```python
from build123d import *

# Parameters (mm, degrees)
SKETCH1_W           = 152.4
SKETCH1_H           = 50.8
BOSS_EXTRUDE1_DEPTH = 6
BOSS_EXTRUDE2_DEPTH = 152.4
SKETCH7_W           = 16.51
SKETCH7_H           = 19.05
SKETCH7_R           = 2
BOSS_EXTRUDE3_DEPTH = 7
FILLET1_R           = 3.175
SKETCH8_R           = 3.025
CUT_EXTRUDE1_DEPTH  = 10


with BuildPart() as part:
    # Sketch1 → Boss-Extrude1 (new body)
    with BuildSketch(Plane.XY):
        Rectangle(SKETCH1_W, SKETCH1_H)
    extrude(amount=BOSS_EXTRUDE1_DEPTH)

    # Sketch5 → Boss-Extrude2 (add)
    with BuildSketch(Plane.ZY.offset(76.2)):
        Polygon((6, 25.4), (24.489687901, 25.4), (6, -25.4), align=None)
    extrude(amount=-BOSS_EXTRUDE2_DEPTH)

    # Sketch7 → Boss-Extrude3 (add)
    # profile 1 of 2: a face of its own
    with BuildSketch(Plane(origin=(0, 0, 0), x_dir=(-1, 0, 0), z_dir=(0, 0, -1))):
        with Locations((-84.455, 0)):
            Rectangle(SKETCH7_W, SKETCH7_H)
        with Locations((-84.455, 0)):
            Circle(SKETCH7_R, mode=Mode.SUBTRACT)
    # profile 2 of 2: a face of its own
    with BuildSketch(Plane(origin=(0, 0, 0), x_dir=(-1, 0, 0), z_dir=(0, 0, -1))):
        with Locations((84.455, 0)):
            Rectangle(SKETCH7_W, SKETCH7_H)
        with Locations((84.455, 0)):
            Circle(SKETCH7_R, mode=Mode.SUBTRACT)
    extrude(amount=-BOSS_EXTRUDE3_DEPTH)

    # Fillet1
    fillet1_edges = [part.edges().sort_by_distance(p)[0] for p in [
        (-76.2, 0, 15.24484395),
        (76.2, 0, 15.24484395),
        (0, 25.4, 24.489687901),
        (0, -25.4, 6),
        (76.2, -9.525, 3.5),
        (92.71, -9.525, 3.5),
        (92.71, 9.525, 3.5),
        (76.2, 9.525, 3.5),
        (-76.2, -9.525, 3.5),
        (-76.2, 9.525, 3.5),
        (-92.71, 9.525, 3.5),
        (-92.71, -9.525, 3.5),
        (76.2, -25.4, 3),
        (-76.2, -25.4, 3),
        (-76.2, 25.4, 12.24484395),
        (76.2, 25.4, 12.24484395),
    ]]
    fillet(fillet1_edges, radius=FILLET1_R)

    # Sketch8 → Cut-Extrude1 (cut)
    with BuildSketch(Plane(origin=(0, -4.899598401, 13.461535972), x_dir=(1, 0, 0), z_dir=(0, -0.3420201433256695, 0.9396926207859082))):
        with Locations(Location((-66.11875, 7.355813283, 0), (0, 0, 270))):
            Circle(SKETCH8_R)
        with Locations(Location((66.11875, 7.355813283, 0), (0, 0, 270))):
            Circle(SKETCH8_R)
    extrude(amount=-CUT_EXTRUDE1_DEPTH, mode=Mode.SUBTRACT)


solid = part.part
```
Could you check a few things on this model? Use its own coordinates, in mm. A direction names the side the tool comes from. Give positions to 0.01 mm unless a question says otherwise; leave off trailing zeros. Order: outer loops, then holes, each group sorted by start corner. A loop starts at its lowest first (then second) coordinate and runs counter-clockwise, first axis right, second up.
Q1. I'm going to push flat-ended pins straight in: P1, Ø5, axis at x = -84.455, y = 0, coming from the +Z side; P2, Ø3.5, axis at x = 86, z = 5, coming from the -Y side (3 decimals); P3, Ø1, axis at x = 67, z = 16, coming from the -Y side. Where does each tip first touch, or does it pass through?
Q2. For faces 4 (the flat face through (85, -9.525, 3)), 5 (the flat face through (85, -3, 7)), 6 (the cylindrical face through (-91.755, 8.62, 3.549)), which set-ups out of +Z, -Z, +X, -X, +Y, -Y let a thin tool reach every point of the face, with its end or its side?
Q3. If I drill on line 1 along X through (y, z) = (-2, 11.25); line 2 along Z through (x, y) = (-57, -7); line 3 along X through (y, z) = (20, 21.75), over which ranges is the centre line in solid material (lowest first)?
Q4. We'd pull the mould along X, two halves only. Please class faces 1 (the flat face through (-76.2, 5, 8)), 2 (the flat face through (-1.022, -0.775, 14.963)), 3 (the flat face through (-66.076, 5.473, 6.595)): +X half, -X half, draft (parallel to the pull), parting line (faces both ways), or undercut.
Q5. Suppose I cut it at A-A, the plane x = 45. Write out the boundary of the cut face in (y, z) (3 decimals).
Solution:
1. P1: stops at z = 7
1. P2: stops at y = -9.525
1. P3: stops at y = 4.81
2. face 4: +Z, -Z, +X, -Y
2. face 5: +Z, +X, +Y, -Y
2. face 6: +Z, -Z, -X, +Y
3. line 1: x = -76.2 to 76.2
3. line 2: z = 0 to 12.7
3. line 3: x = -75.05 to 75.05
4. face 1: -X half
4. face 2: draft
4. face 3: undercut
5. outline: (-25.4, 0) - (25.4, 0) - (25.4, 19.955) arc R3.175 ccw to (21.139, 22.939) - (-23.311, 6.76) arc R3.175 ccw to (-25.4, 3.777) - close
